Autodesk Inventor part; units mm, degrees
ref_plane "YZ Plane" through (0, 0, 0) normal (1, 0, 0) x (0, 1, 0)
ref_plane "XZ Plane" through (0, 0, 0) normal (0, 1, 0) x (-1, 0, 0)
ref_plane "XY Plane" through (0, 0, 0) normal (0, 0, 1) x (1, 0, 0)
sketch "Sketch36" plane through (0, 0, 0) normal (0, 0, 1) x (1, 0, 0)
  arc A0 (0, -5.7547) -> (0, 5.7547) centre (0, 0) ccw
  arc A1 (-12.7, 5.7547) -> (-12.7, -5.7547) centre (-12.7, 0) ccw
  line L0 (-12.7, 5.7547) -> (0, 5.7547)
  line L1 (-12.7, -5.7547) -> (0, -5.7547)
  circle A2 centre (-12.7, 0) radius 1.1906
  circle A3 centre (0, 0) radius 1.1906
  dimension "d158" = 11.5094
  dimension "d160" = 12.7
  dimension "d162" = 2.3813
  dimension "d163" = 2.3813
  dimension "d176" = 5.7547
extrude "Extrusion36" add sketch "Sketch36" along normal blind 1.5875
chamfer "Chamfer2" distance 0.7937 angle 45 2 edges at (-13.8906, 0, 1.5875) (-1.1906, 0, 1.5875)
properties part number "arm-top"
CAD build for the part. Positions are in the model's coordinates, mm. Give positions to 0.01 mm unless a question says otherwise; leave off trailing zeros. Order: outer loops, then holes, each group sorted by start corner. A loop starts at its lowest first (then second) coordinate and runs counter-clockwise, first axis right, second up. Notation, with made-up numbers: (4, -27) - (48, -27) arc R16 ccw to (48, -17) - close; hole circle Ø5 at (65.25, 60). An arc over 180 degrees is marked (long way). Write each question's results on one line, items separated by ' | '.
1. Saw through at D-D on y = 3. List the corners of the cut face in (x, z).
Calculated:
outline: (-17.61, 0) - (4.91, 0) - (4.91, 1.59) - (-17.61, 1.59) - close
2. Pin check, flat tip, straight feed: pin 1 (1 mm diameter, centred on x = 3, y = 3, fed in from -Z). Stop position of the tip, or through.
Calculated:
pin 1: stops at z = 0
3. Pull direction X, two halves, no side cores. Call faces 1 (the face through (5.753, 0.127, 0.783)), 2 (the face through (-6, 5.755, 1)), 3 (the face through (-18.453, -0.127, 0.783)), 4 (the face through (-11.6, 0.46, 0.39)): released by +X, released by -X, zero draft, split by the parting line, or undercut.
Calculated:
face 1: released by +X | face 2: zero draft | face 3: released by -X | face 4: undercut
4. Saw through at B-B on z = 0.5. List the corners of the cut face in (x, y), and give its area (3 significant figures).
Calculated:
outline: (-12.7, -5.75) - (0, -5.75) arc R5.75 ccw to (0, 5.75) - (-12.7, 5.75) arc R5.75 ccw to start; hole circle Ø2.38 at (-12.7, 0); hole circle Ø2.38 at (0, 0) | area: 241 mm2
5. Saw through at C-C on y = 5.25. List the corners of the cut face in (x, z).
Calculated:
outline: (-15.06, 0) - (2.36, 0) - (2.36, 1.59) - (-15.06, 1.59) - close
6. Saw through at A-A on y = 0. List the corners of the cut face in (x, z).
Calculated:
outline: (-18.45, 0) - (-13.89, 0) - (-13.89, 0.79) - (-14.68, 1.59) - (-18.45, 1.59) - close; (-11.51, 0) - (-1.19, 0) - (-1.19, 0.79) - (-1.98, 1.59) - (-10.72, 1.59) - (-11.51, 0.79) - close; (1.19, 0) - (5.75, 0) - (5.75, 1.59) - (1.98, 1.59) - (1.19, 0.79) - close
7. Probe L1, parallel to Y at x = 0, z = 0.2; L2, parallel to Y at x = -14.75, z = 0.6; L3, parallel to Y at x = -15.25, z = 0.9. List the from-to ranges inside material, lowest first. Write a range as from..to.
Calculated:
L1: y = -5.75..-1.19, 1.19..5.75 | L2: y = -5.38..5.38 | L3: y = -5.16..5.16
